For this review, take the finished solid that the model builds, in its own axes (mm). A direction names the side the tool comes from. Coordinates: 2 decimals unless noted, no trailing zeros. Write each loop counter-clockwise with the first axis right and the second up, starting at its lowest first coordinate (ties: lowest second). Pieces come first, ordered by that corner, then holes.
```python
from build123d import *

# Parameters (mm, degrees)
CROQUIS1_W              = 14.2
CROQUIS1_H              = 32
SALIENTE_EXTRUIR1_DEPTH = 1.6
CROQUIS2_R              = 1.5
CORTAR_EXTRUIR1_DEPTH   = 18.57754249
SALIENTE_EXTRUIR2_DEPTH = 10
CROQUIS4_R              = 1.5
CROQUIS4_W              = 0.5
CROQUIS4_H              = 3.5
CORTAR_EXTRUIR2_DEPTH   = 2
CHAFL_N1_SIZE           = 1
REDONDEO1_R             = 1.5
CROQUIS5_W              = 7
CROQUIS5_H              = 7
SALIENTE_EXTRUIR3_DEPTH = 5


with BuildPart() as part:
    # Croquis1 → Saliente-Extruir1 (new body)
    with BuildSketch(Plane.XY):
        Rectangle(CROQUIS1_W, CROQUIS1_H)
    extrude(amount=SALIENTE_EXTRUIR1_DEPTH)

    # Croquis2 → Cortar-Extruir1 (cut, through all)
    with BuildSketch(Plane.XY.offset(1.6)):
        with Locations((-0.1, -8.35)):
            Circle(CROQUIS2_R)
    extrude(amount=-CORTAR_EXTRUIR1_DEPTH, mode=Mode.SUBTRACT)

    # Croquis3 → Saliente-Extruir2 (add)
    with BuildSketch(Plane.XY.offset(1.6)):
        Polygon((-5, 16), (3.7, 16), (5, 14.7), (5, 11.7), (3.7, 10.4), (-5, 10.4), align=None)
    extrude(amount=SALIENTE_EXTRUIR2_DEPTH)

    # Croquis4 → Cortar-Extruir2 (cut)
    with BuildSketch(Plane.XY.offset(11.6)):
        Polygon((-5, 10.4), (3.7, 10.4), (5, 11.7), (5, 14.7), (3.7, 16), (-5, 16), align=None)
        with Locations((-2.25, 13.2)):
            Circle(CROQUIS4_R, mode=Mode.SUBTRACT)
        with Locations((2.25, 13.2)):
            Circle(CROQUIS4_R, mode=Mode.SUBTRACT)
        with Locations((0, 13.2)):
            Rectangle(CROQUIS4_W, CROQUIS4_H, mode=Mode.SUBTRACT)
    extrude(amount=-CORTAR_EXTRUIR2_DEPTH, mode=Mode.SUBTRACT)

    # Chaflán1
    chafl_n1_edges = [part.edges().sort_by_distance(p)[0] for p in [
        (4.35, 15.35, 9.6),
        (5, 13.2, 9.6),
        (4.35, 11.05, 9.6),
        (-0.65, 10.4, 9.6),
        (-5, 13.2, 9.6),
        (-0.65, 16, 9.6),
    ]]
    chamfer(chafl_n1_edges, length=CHAFL_N1_SIZE)

    # Redondeo1
    redondeo1_edges = [part.edges().sort_by_distance(p)[0] for p in [
        (-3.75, 13.2, 11.6),
        (0.75, 13.2, 11.6),
    ]]
    fillet(redondeo1_edges, radius=REDONDEO1_R)

    # Croquis5 → Saliente-Extruir3 (add)
    with BuildSketch(Plane(origin=(0, 0, 0), x_dir=(-1, 0, 0), z_dir=(0, 0, -1))):
        with Locations((3.1, 0.5)):
            Rectangle(CROQUIS5_W, CROQUIS5_H)
    extrude(amount=SALIENTE_EXTRUIR3_DEPTH)


solid = part.part
```
Q1. Clearance check with flat-ended pins moving along their axes: pin 1 Ø4 at (y, z) = (5.5, -3) entering from -X; pin 2 Ø1.1 at (x, y) = (1, 13.5) entering from +Z; pin 3 Ø0.6 at (x, z) = (0, 11) entering from -Y; pin 4 Ø2.5 at (x, y) = (-0.1, -8.35) entering from +Z. State where each tip first meets the part, or that it passes through.
Ans:
pin 1: stops at x = -6.6
pin 2: stops at z = 11.41
pin 3: stops at y = 11.45
pin 4: passes through
Q2. Add section A-A (y = -8.35). State the section outline as (x, z) points, then the cut area to 3 significant figures.
Ans:
outline: (-7.1, 0) - (-1.6, 0) - (-1.6, 1.6) - (-7.1, 1.6) - close; (1.4, 0) - (7.1, 0) - (7.1, 1.6) - (1.4, 1.6) - close
area: 17.9 mm2
Q3. Add section C-C (z = 1). State the section outline as (x, y) points.
Ans:
outline: (-7.1, -16) - (7.1, -16) - (7.1, 16) - (-7.1, 16) - close; hole circle Ø3 at (-0.1, -8.35)
Q4. Draft analysis for pull direction X (two halves, no side actions). For faces 6 (the cylindrical face through (-1.444, 14.465, 9.854)), 7 (the flat face through (-0.25, 13, 11)), 8 (the flat face through (4.07, 11.31, 8.98)), 9 (the flat face through (-1, 10.4, 5)), state which applies: +X half, -X half, draft (parallel to the pull), parting line (faces both ways), or undercut.
Ans:
face 6: undercut
face 7: undercut
face 8: +X half
face 9: draft
Q5. Tool access review of faces 1 (the flat face through (-5, 13, 5)), 2 (the flat face through (4.3, 15.4, 5.1)), 3 (the flat face through (5, 13, 5)), 4 (the flat face through (4.4, 11.1, 5.1)), 5 (the flat face through (-3, 4, -2)): name each direction out of +Z, -Z, +X, -X, +Y, -Y from which nothing blocks a thin tool from reaching the whole face with its end or side.
Ans:
face 1: +Z, -X, +Y, -Y
face 2: +Z, +X, +Y
face 3: +Z, +X, +Y, -Y
face 4: +Z, +X, -Y
face 5: -Z, +X, -X, +Y
Q6. Add section D-D (y = 1). State the section outline as (x, z) points.
Ans:
outline: (-7.1, 0) - (-6.6, 0) - (-6.6, -5) - (0.4, -5) - (0.4, 0) - (7.1, 0) - (7.1, 1.6) - (-7.1, 1.6) - close
Q7. Add section B-B (x = 2.25). State the section outline as (y, z) points, then the cut area to 3 significant figures.
Ans:
outline: (-16, 0) - (16, 0) - (16, 8.6) - (15, 9.6) - (14.7, 9.6) - (14.7, 10.1) arc R1.5 ccw to (11.7, 10.1) - (11.7, 9.6) - (11.4, 9.6) - (10.4, 8.6) - (10.4, 1.6) - (-16, 1.6) - close
area: 100 mm2
Q8. For probe 1 along Y at (x, z) = (-0.1, 1); probe 2 along Z at (x, y) = (5.5, -9); probe 3 along Y at (x, z) = (-1, 7), list the stretches that pass through material, from the lowest coordinate up.
Ans:
probe 1: y = -16 to -9.85, -6.85 to 16
probe 2: z = 0 to 1.6
probe 3: y = 10.4 to 16
